Autodesk Inventor part; units mm, degrees
ref_plane "YZ Plane" through (0, 0, 0) normal (1, 0, 0) x (0, 1, 0)
ref_plane "XZ Plane" through (0, 0, 0) normal (0, 1, 0) x (-1, 0, 0)
ref_plane "XY Plane" through (0, 0, 0) normal (0, 0, 1) x (1, 0, 0)
sketch "Sketch1" plane through (0, 0, 0) normal (0, 1, 0) x (-1, 0, 0)
  line L0 (7.9868, 9.2079) -> (-2.0132, 9.2079)
  line L1 (-2.0132, 9.2079) -> (-2.0132, -10.7921)
  line L2 (-2.0132, -10.7921) -> (7.9868, -10.7921)
  line L3 (7.9868, -10.7921) -> (7.9868, 9.2079)
  point P0 (0, 0)
  dimension "height" = 20
  dimension "width" = 10
extrude "Extrusion1" add sketch "Sketch1" along normal blind 10
sketch "Sketch2" plane through (0, 10, 0) normal (0, 1, 0) x (1, 0, 0)
  line L0 (-7.9868, 10.7921) -> (-7.9868, -9.2079) construction
  line L1 (-7.9868, 0.7921) -> (2.0132, 0.7921) construction
  line L2 (2.0132, -9.2079) -> (2.0132, 10.7921) construction
  line L3 (-7.9868, -9.2079) -> (2.0132, -9.2079) construction
  line L4 (-2.9868, -9.2079) -> (-2.9868, 10.7921) construction
  line L5 (2.0132, 10.7921) -> (-7.9868, 10.7921) construction
  circle A0 centre (-2.9868, 0.7921) radius 4
  point P0 (0, 0)
  dimension "hole" = 8
extrude "Extrusion3" cut sketch "Sketch2" against normal blind 5
sketch "Sketch3" plane through (0, 10, 0) normal (0, 1, 0) x (1, 0, 0)
  circle A0 centre (-5.4186, 8.4854) radius 1.4583
  point P0 (0, 0)
extrude "Extrusion4" cut sketch "Sketch3" against normal blind 2
equation "\"width\" = 0.5 * height"
For this review, take the finished solid that the model builds, in its own axes (mm). A direction names the side the tool comes from. Round coordinates to 2 decimals unless told otherwise and drop trailing zeros. Loops run counter-clockwise (first coordinate to the right, second up) from the corner with the lowest first, then second, coordinate; pieces in that order, holes last. Notation, with made-up numbers: (58.5, -27.75) - (90.5, -27.75) arc R30 ccw to (90.5, 1.25) - close; hole circle Ø4 at (-21, 19). An arc over 180 degrees is marked (long way). One line per question, with ' | ' between items.
Q1. Tool access review of faces 1 (the flat face through (-3, 5, -10.792)), 2 (the flat face through (-3, 5, -1)): name each direction out of +Z, -Z, +X, -X, +Y, -Y from which nothing blocks a thin tool from reaching the whole face with its end or side.
Taken from the geometry:
face 1: -Z, +X, -X, +Y, -Y | face 2: +Y
Q2. Take a section at B-B (z = -2.5). Give the boundary of the cut face in (x, y), and give its area (3 significant figures).
Taken from the geometry:
outline: (-7.99, 0) - (2.01, 0) - (2.01, 10) - (0.63, 10) - (0.63, 5) - (-6.6, 5) - (-6.6, 10) - (-7.99, 10) - close | area: 63.8 mm²
Q3. Take a section at C-C (y = 5.75). Give the boundary of the cut face in (x, z), and give its area (3 significant figures).
Taken from the geometry:
outline: (-7.99, -10.79) - (2.01, -10.79) - (2.01, 9.21) - (-7.99, 9.21) - close; hole circle Ø8 at (-2.99, -0.79) | area: 150 mm²
Q4. For pin 1 (2.5 mm diameter, centred on x = -1.5, z = 0, fed in from +Y); pin 2 (2.5 mm diameter, centred on x = -5.42, z = -8.49, fed in from +Y), all flat-tipped, find the tip position at first contact; note any pin that passes through.
Taken from the geometry:
pin 1: stops at y = 5 | pin 2: stops at y = 8
Q5. For line 1 along Z through (x, y) = (-4.5, 5.25); line 2 along Y through (x, z) = (-6, -2.75); line 3 along Z through (x, y) = (-1, 5.25), list the stretches that pass through material, from the lowest coordinate up. Write a range as [from, to].
Taken from the geometry:
line 1: z = [-10.79, -4.49], [2.91, 9.21] | line 2: y = [0, 5] | line 3: z = [-10.79, -4.26], [2.68, 9.21]
Q6. Take a section at A-A (x = -5.5). Give the boundary of the cut face in (y, z).
Taken from the geometry:
outline: (0, -10.79) - (10, -10.79) - (10, -9.94) - (8, -9.94) - (8, -7.03) - (10, -7.03) - (10, -3.9) - (5, -3.9) - (5, 2.32) - (10, 2.32) - (10, 9.21) - (0, 9.21) - close
Q7. The part is to be moulded in two halves that separate along X. For faces 3 (the cylindrical face through (-6.576, 9.014, -7.598)), 4 (the flat face through (-3, 0, -1)), 5 (the flat face through (-5, 8, -9)), 6 (the flat face through (2.013, 5, -1)), say which applies: released by +X, released by -X, zero draft, split by the parting line, or undercut.
Taken from the geometry:
face 3: undercut | face 4: zero draft | face 5: undercut | face 6: released by +X
Q8. Take a section at D-D (x = -4.5). Give the boundary of the cut face in (y, z).
Taken from the geometry:
outline: (0, -10.79) - (10, -10.79) - (10, -9.62) - (8, -9.62) - (8, -7.35) - (10, -7.35) - (10, -4.49) - (5, -4.49) - (5, 2.91) - (10, 2.91) - (10, 9.21) - (0, 9.21) - close
